Build history of the part. All positions in model axes, mm. A direction names the side the tool comes from. Round coordinates to 2 decimals unless told otherwise and drop trailing zeros. Write each loop counter-clockwise with the first axis right and the second up, starting at its lowest first coordinate (ties: lowest second). Pieces come first, ordered by that corner, then holes.
Item 1: Drop flat-ended pins along their axis: pin 1 Ø1.5 at (x, z) = (-7.5, 0) entering from +Y; pin 2 Ø3 at (x, y) = (-6, 1) entering from +Z; pin 3 Ø1.5 at (x, z) = (-3, -0.5) entering from -Y. Give the stop position or say it passes through.
Item 2: Mould opens along Y. For faces 1 (the flat face through (-10.956, 0.631, 1.565)), 2 (the flat face through (-11.449, -1, 2)), 3 (the cylindrical face through (-9.894, -2.685, 1.047)) say: +Y half, -Y half, draft (parallel to the pull), parting line (faces both ways), or undercut.
Item 3: Band-saw the part on B-B, the plane x = 3.5. Write the cut outline in (y, z), then the cut area to 3 significant figures.
Item 4: Wall check: probe 1 along X at (y, z) = (0.4, -0.6); probe 2 along X at (y, z) = (0.25, -1.85); probe 3 along Z at (x, y) = (2, 0.15). Give the ranges that are in metal, low to high.
Item 5: 3-axis set-ups, long thin cutter, end or side, ignore diameter. For faces 4 (the flat face through (-8.449, -1, 2)), 5 (the flat face through (-10.96, 0.65, -0.65)), 6 (the flat face through (8.831, 0, 0)): which of +Z, -Z, +X, -X, +Y, -Y reach the whole face in a straight line?
Item 6: Band-saw the part on A-A, the plane x = -9. Write the cut outline in (y, z).
```python
from build123d import *

# Parameters (mm, degrees)
FILLET2_R          = 0.15
CUT_EXTRUDE1_DEPTH = 1


with BuildPart() as part:
    # Sketch1 → Revolve2 (revolve)
    with BuildSketch(Plane(origin=(0, 0, 0), x_dir=(1, 0, 0), z_dir=(0, 1, 0))):
        Polygon((-11.44921875, 2.298828125), (-11.44921875, -0.451171875), (8.83128125, -0.451171875), (8.83128125, 0.768328125), (8.55078125, 1.048828125), (-8.44921875, 1.048828125), (-8.44921875, 2.298828125), align=None)
    revolve(axis=Axis((-15.512494932, 0, 0.451171875), (1, 0, 0)))

    # Fillet2
    fillet2_edges = [part.edges().sort_by_distance(p)[0] for p in [
        (-11.44921875, 0, 3.201171875),
        (-8.44921875, 0, 1.951171875),
    ]]
    fillet(fillet2_edges, radius=FILLET2_R)

    # Sketch3 → Cut-Extrude1 (cut)
    with BuildSketch(Plane.ZY.offset(11.44921875)):
        Polygon((1.190118859, -1.280035428), (1.929188565, -7.0854e-05), (1.190241581, 1.279964574), (-0.287775109, 1.280035428), (-1.026844815, 7.0854e-05), (-0.287897831, -1.279964574), align=None)
    extrude(amount=-CUT_EXTRUDE1_DEPTH, mode=Mode.SUBTRACT)


solid = part.part
```
Results:
1. pin 1: stops at y = 1.5
1. pin 2: stops at z = 1.95
1. pin 3: stops at y = -1.49
2. face 1: undercut
2. face 2: draft
2. face 3: parting line
3. outline: circle Ø3 at (0, 0.45)
3. area: 7.07 mm2
4. probe 1: x = -10.45 to 8.83
4. probe 2: x = -11.45 to -8.45
4. probe 3: z = -1.04 to 1.94
5. face 4: +X
5. face 5: -X
5. face 6: +Z, -Z, +X, +Y, -Y
6. outline: circle Ø5.5 at (0, 0.45)
